Source: CAD feature listing. Evaluate the final solid. Frame: model axes, mm. Round coordinates to 2 decimals unless told otherwise and drop trailing zeros. Write each loop counter-clockwise with the first axis right and the second up, starting at its lowest first coordinate (ties: lowest second). Pieces come first, ordered by that corner, then holes. Notation, with made-up numbers: M 45.25,66.25 L 75.25,66.25 A23 cw 75.25,84.25 Z; hole C 7.25,-33 d9. An arc over 180 degrees is marked long. Answer in a Markdown table with one row per item.
from build123d import *

# Parameters (mm, degrees)
BOSS_EXTRUDE1_DEPTH          = 2.65684
F_10_0_1935_DIAMETER_HOLE1_D = 4.9149
FILLET1_R                    = 3.175


with BuildPart() as part:
    # Sketch1 → Boss-Extrude1 (new body)
    with BuildSketch(Plane(origin=(0, 0, 0), x_dir=(1, 0, 0), z_dir=(0, 1, 0))):
        Polygon((127, 88.9), (127, 127), (88.9, 127), (0, 127), (0, 0), (38.1, 0), (38.1, 38.1), (88.9, 88.9), align=None)
    extrude(amount=BOSS_EXTRUDE1_DEPTH)

    # #10 (0.1935) Diameter Hole1 (through all)
    with Locations(Plane(origin=(0, 2.65684, 0), x_dir=(1, 0, 0), z_dir=(0, 1, 0))):
        with Locations((114.3, 107.95), (66.675, 107.95), (19.05, 107.95), (19.05, 60.325), (19.05, 12.7)):
            Hole(F_10_0_1935_DIAMETER_HOLE1_D / 2)

    # Fillet1
    fillet1_edges = [part.edges().sort_by_distance(p)[0] for p in [
        (127, 1.32842, -88.9),
        (38.1, 1.32842, 0),
        (0, 1.32842, 0),
        (0, 1.32842, -127),
        (127, 1.32842, -127),
    ]]
    fillet(fillet1_edges, radius=FILLET1_R)


solid = part.part
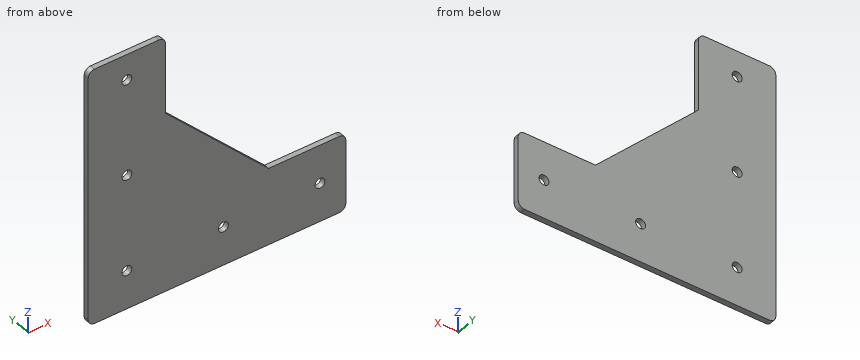
Q1. Section D-D (y = 1.6). Return loops of the section in (x, z) (3 decimals).
Solutions:
| item | result |
|---|---|
| outline | M 0,-123.825 A3.175 ccw 3.175,-127 L 123.825,-127 A3.175 ccw 127,-123.825 L 127,-92.075 A3.175 ccw 123.825,-88.9 L 88.9,-88.9 L 38.1,-38.1 L 38.1,-3.175 A3.175 ccw 34.925,0 L 3.175,0 A3.175 ccw 0,-3.175 Z; hole C 19.05,-107.95 d4.915; hole C 19.05,-60.325 d4.915; hole C 19.05,-12.7 d4.915; hole C 66.675,-107.95 d4.915; hole C 114.3,-107.95 d4.915 |
Q2. Section A-A (z = -12.7). Return loops of the section in (x, y).
Solutions:
| item | result |
|---|---|
| outline | M 0,0 L 16.59,0 L 16.59,2.66 L 0,2.66 Z; M 21.51,0 L 38.1,0 L 38.1,2.66 L 21.51,2.66 Z |
Q3. Material intervals for probe 1 along Z at (x, y) = (19.05, 1.35); probe 2 along X at (y, z) = (1.3, -107.95); probe 3 along X at (y, z) = (0.6, -28.5), sorted ascending.
Solutions:
| item | result |
|---|---|
| probe 1 | z = -127 to -110.41, -105.49 to -62.78, -57.87 to -15.16, -10.24 to 0 |
| probe 2 | x = 0 to 16.59, 21.51 to 64.22, 69.13 to 111.84, 116.76 to 127 |
| probe 3 | x = 0 to 38.1 |
Q4. Contact query for flat-ended pins moving along their axis: pin 1 Ø3 at (x, z) = (19.05, -12.7) entering from -Y; pin 2 Ø0.8 at (x, y) = (104, 1.5) entering from +Z; pin 3 Ø1.3 at (y, z) = (0.5, -26.5) entering from +X. Output: stop coordinate, or through.
Solutions:
| item | result |
|---|---|
| pin 1 | passes through |
| pin 2 | stops at z = -88.9 |
| pin 3 | stops at x = 38.1 |
Q5. Section B-B (x = 19.05). Return loops of the section in (y, z).
Solutions:
| item | result |
|---|---|
| outline | M 0,-127 L 2.66,-127 L 2.66,-110.41 L 0,-110.41 Z; M 0,-105.49 L 2.66,-105.49 L 2.66,-62.78 L 0,-62.78 Z; M 0,-57.87 L 2.66,-57.87 L 2.66,-15.16 L 0,-15.16 Z; M 0,-10.24 L 2.66,-10.24 L 2.66,0 L 0,0 Z |
Q6. Section C-C (z = -107.95). Return loops of the section in (x, y), and give its area (3 significant figures).
Solutions:
| item | result |
|---|---|
| outline | M 0,0 L 16.59,0 L 16.59,2.66 L 0,2.66 Z; M 21.51,0 L 64.22,0 L 64.22,2.66 L 21.51,2.66 Z; M 69.13,0 L 111.84,0 L 111.84,2.66 L 69.13,2.66 Z; M 116.76,0 L 127,0 L 127,2.66 L 116.76,2.66 Z |
| area | 298 mm2 |
